For this review, take the finished solid that the model builds, in its own axes (mm). A direction names the side the tool comes from. Coordinates: 2 decimals unless noted, no trailing zeros. Order: outer loops, then holes, each group sorted by start corner. A loop starts at its lowest first (then second) coordinate and runs counter-clockwise, first axis right, second up. Notation, with made-up numbers: (56, -32.5) - (115, -32.5) arc R33 ccw to (115, 0.5) - close; hole circle Ø1 at (-26.75, 8). An arc over 180 degrees is marked (long way). One line per item, written item: value. Start each with the question number.
(1) Consider section A-A on x = 0. Write out the cut boundary in (y, z).
(2) Mouldability with a two-part tool opening along X and no side actions: class faces 6 (the flat face through (36.8, 30, 0)), 7 (the flat face through (-38, 20.808, 0)), 8 (the flat face through (0, 30, 36.8)) as released by +X, released by -X, zero draft, split by the parting line, or undercut.
(3) To check wall thickness, follow line 1 along Z through (x, y) = (-6, 70); line 2 along X through (y, z) = (24.5, -21); line 3 along X through (y, z) = (59.5, -15.5). State the ranges of each line that lie inside material, in increasing order.
(4) Consider section B-B on z = 0. Write out the cut boundary in (x, y).
(5) Clearance check with flat-ended pins moving along their axes: pin 1 (3.5 mm diameter, centred on x = -7, y = 30, fed in from -Z); pin 2 (20 mm diameter, centred on x = 5, y = 27, fed in from -Z); pin 3 (2.5 mm diameter, centred on x = -6.5, y = 30, fed in from +Z); pin 4 (8 mm diameter, centred on y = 44, z = 14.5, fed in from +X). State where each tip first meets the part, or that it passes through.
(6) Consider section D-D on y = 16. Write out the cut boundary in (x, z).
(7) For faces 1 (the flat face through (0, 20.808, 38)), 2 (the flat face through (-38, 39.192, 0)), 3 (the flat face through (0, 39.192, -38)), 4 (the flat face through (32, 0, 6)), 5 (the flat face through (38, 39.192, 0)), list the 3-axis set-ups (+Z, -Z, +X, -X, +Y, -Y) from which the entire face can be reached by the end or side of a thin tool; tool diameter is ignored.
(8) Consider section C-C on y = 34.5. Write out the cut boundary in (x, z), then the cut area to 3 significant figures.
```python
from build123d import *

# Parameters (mm, degrees)
SKETCH2_R           = 39.3
SKETCH2_R_2         = 32.4
BOSS_EXTRUDE1_DEPTH = 100
CUT_EXTRUDE1_START  = 39.3
CUT_EXTRUDE1_DEPTH  = 2.5
SKETCH4_R           = 1.1
CUT_EXTRUDE2_DEPTH  = 3
CIRPATTERN1_COUNT   = 4
CHAMFER1_SIZE       = 5.8
CHAMFER1_SIZE2      = 4.4


with BuildPart() as part:
    # Sketch2 → Boss-Extrude1 (new body)
    with BuildSketch(Plane(origin=(0, 0, 0), x_dir=(1, 0, 0), z_dir=(0, 1, 0))):
        with Locations(Location((0, 0, 0), (0, 0, 270))):
            Circle(SKETCH2_R)
        with Locations(Location((0, 0, 0), (0, 0, 270))):
            Circle(SKETCH2_R_2, mode=Mode.SUBTRACT)
    extrude(amount=BOSS_EXTRUDE1_DEPTH)

    # Sketch3 → Cut-Extrude1 (cut)
    with BuildSketch(Plane.XY.offset(CUT_EXTRUDE1_START)):
        with BuildLine():
            Line((9.192388155, 39.192388155), (-9.192388155, 39.192388155))
            ThreePointArc((-9.192388155, 39.192388155), (-13, 30), (-9.192388155, 20.807611845))
            Line((-9.192388155, 20.807611845), (9.192388155, 20.807611845))
            ThreePointArc((9.192388155, 20.807611845), (13, 30), (9.192388155, 39.192388155))
        make_face()
    cut_extrude1 = extrude(amount=-CUT_EXTRUDE1_DEPTH, mode=Mode.SUBTRACT)

    # Sketch4 → Cut-Extrude2 (cut)
    with BuildSketch(Plane.XY.offset(36.8)):
        with Locations((7, 30)):
            Circle(SKETCH4_R)
        with Locations((-7, 30)):
            Circle(SKETCH4_R)
    cut_extrude2 = extrude(amount=-CUT_EXTRUDE2_DEPTH, mode=Mode.SUBTRACT)

    # CirPattern1: Cut-Extrude1, Cut-Extrude2 ×4 about axis
    cirpattern1_axis = Axis((0, 0, 0), (0, 1, 0))
    add([cut_extrude1.rotate(cirpattern1_axis, i * 360 / CIRPATTERN1_COUNT) for i in range(1, CIRPATTERN1_COUNT)], mode=Mode.SUBTRACT)
    add([cut_extrude2.rotate(cirpattern1_axis, i * 360 / CIRPATTERN1_COUNT) for i in range(1, CIRPATTERN1_COUNT)], mode=Mode.SUBTRACT)

    # Chamfer1
    chamfer1_edges = [part.edges().sort_by_distance(p)[0] for p in [
        (0, 100, -32.4),
    ]]
    chamfer1_side = [part.faces().sort_by_distance(p)[0] for p in [
        (0, 100, -38.18842814),
    ]]
    chamfer(chamfer1_edges, length=CHAMFER1_SIZE, length2=CHAMFER1_SIZE2, reference=chamfer1_side[0])


solid = part.part
```
Geometry check:
1. outline: (0, -39.3) - (20.81, -39.3) - (20.81, -36.8) - (39.19, -36.8) - (39.19, -39.3) - (100, -39.3) - (100, -38.2) - (95.6, -32.4) - (0, -32.4) - close; (0, 32.4) - (95.6, 32.4) - (100, 38.2) - (100, 39.3) - (39.19, 39.3) - (39.19, 36.8) - (20.81, 36.8) - (20.81, 39.3) - (0, 39.3) - close
2. face 6: released by +X
2. face 7: zero draft
2. face 8: undercut
3. line 1: z = -38.84 to -31.84, 31.84 to 38.84
3. line 2: x = -33.22 to -24.67, 24.67 to 33.22
3. line 3: x = -36.11 to -28.45, 28.45 to 36.11
4. outline: (-39.3, 0) - (-32.4, 0) - (-32.4, 95.6) - (-38.2, 100) - (-39.3, 100) - (-39.3, 39.19) - (-36.8, 39.19) - (-36.8, 20.81) - (-39.3, 20.81) - close; (32.4, 0) - (39.3, 0) - (39.3, 20.81) - (36.8, 20.81) - (36.8, 39.19) - (39.3, 39.19) - (39.3, 100) - (38.2, 100) - (32.4, 95.6) - close
5. pin 1: stops at z = -36.8
5. pin 2: stops at z = -39.3
5. pin 3: stops at z = 36.8
5. pin 4: stops at x = 37.87
6. outline: circle Ø78.6 at (0, 0); hole circle Ø64.8 at (0, 0)
7. face 1: +Z
7. face 2: -X
7. face 3: -Z
7. face 4: +Z, -Z, +X, -X, -Y
7. face 5: +X
8. outline: (-37.36, -12.2) arc R39.3 ccw to (-12.2, -37.36) - (-12.2, -36.8) - (12.2, -36.8) - (12.2, -37.36) arc R39.3 ccw to (37.36, -12.2) - (36.8, -12.2) - (36.8, 12.2) - (37.36, 12.2) arc R39.3 ccw to (12.2, 37.36) - (12.2, 36.8) - (-12.2, 36.8) - (-12.2, 37.36) arc R39.3 ccw to (-37.36, 12.2) - (-36.8, 12.2) - (-36.8, -12.2) - close; hole circle Ø64.8 at (0, 0)
8. area: 1,370 mm^2
